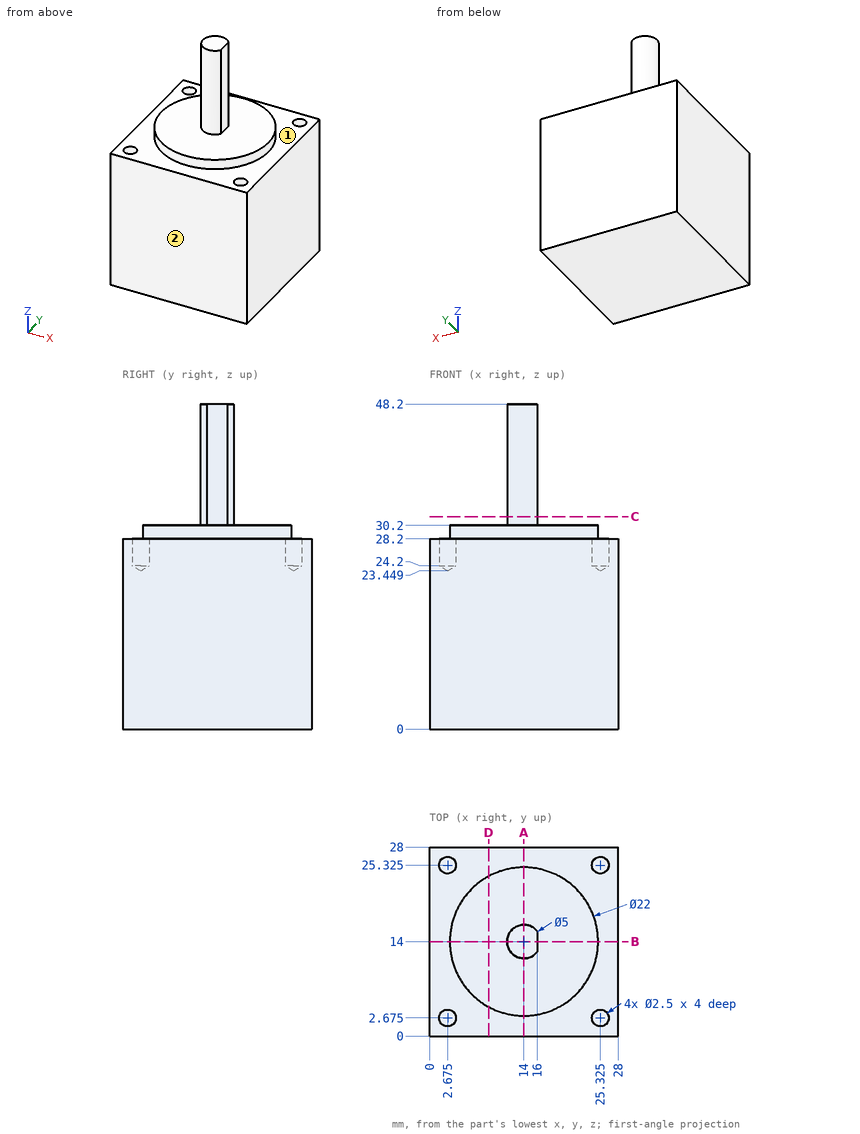
Here's the drawing with two shaded views (mm, measured from the low corner). I have some questions. A direction names the side the tool comes from. Round coordinates to 2 decimals unless told otherwise and drop trailing zeros. Loops run counter-clockwise (first coordinate to the right, second up) from the corner with the lowest first, then second, coordinate; pieces in that order, holes last. Notation, with made-up numbers: (-9.5, 86) - (44.5, 86) arc R12 ccw to (44.5, 109) - close; hole circle Ø6 at (-15.75, -18). An arc over 180 degrees is marked (long way). Use CSV: the item, a comma, the result in double quotes. Start each with the question number.
1) Please list where these lines run through material, in increasing order: probe 1 along Z at (x, y) = (9.75, 10.5); probe 2 along Z at (x, y) = (15, 3); probe 3 along X at (y, z) = (14, 41.5). Write a range as [from, to].
2) If we section it at A-A on x = 14: Write out the boundary of the cut face in (y, z), plus the area to 3 significant figures.
3) For pin 1 Ø3 at (x, y) = (25.325, 2.675) entering from +Z; pin 2 Ø1.5 at (x, z) = (12.5, 34) entering from +Y (3 decimals); pin 3 Ø4 at (x, z) = (11, 32.5) entering from -Y, each with a flat end and sliding along its axis, tell me the tip position at first contact or that it passes through.
4) For the marked faces 1 and 2, which set-ups out of +Z, -Z, +X, -X, +Y, -Y let a thin tool reach every point of the face, with its end or its side?
5) If we section it at C-C on z = 31.5: Write out the boundary of the cut face in (x, y), plus the area to 3 significant figures.
6) If we section it at D-D on x = 8.75: Write out the boundary of the cut face in (y, z).
7) If we section it at B-B on y = 14: Write out the boundary of the cut face in (x, z).
Geometry results:
1,probe 1,"z = [0, 30.2]"
1,probe 2,"z = [0, 28.2]"
1,probe 3,"x = [11.5, 16]"
2,outline,"(0, 0) - (28, 0) - (28, 28.2) - (25, 28.2) - (25, 30.2) - (16.5, 30.2) - (16.5, 48.2) - (11.5, 48.2) - (11.5, 30.2) - (3, 30.2) - (3, 28.2) - (0, 28.2) - close"
2,area,"924 mm2"
3,pin 1,"stops at z = 28.2"
3,pin 2,"stops at y = 16.385"
3,pin 3,"stops at y = 11.71"
4,face 1,"+Z"
4,face 2,"+Z, -Z, +X, -X, -Y"
5,outline,"(16, 12.5) - (16, 15.5) arc R2.5 ccw (long way) to start"
5,area,"18.6 mm2"
6,outline,"(0, 0) - (28, 0) - (28, 28.2) - (23.67, 28.2) - (23.67, 30.2) - (4.33, 30.2) - (4.33, 28.2) - (0, 28.2) - close"
7,outline,"(0, 0) - (28, 0) - (28, 28.2) - (25, 28.2) - (25, 30.2) - (16, 30.2) - (16, 48.2) - (11.5, 48.2) - (11.5, 30.2) - (3, 30.2) - (3, 28.2) - (0, 28.2) - close"
